For this review, use the dimensioned drawing (mm, ordinates from the lowest corner) and the shaded views. A direction names the side the tool comes from. Give positions to 0.01 mm unless a question says otherwise; leave off trailing zeros. Write each loop counter-clockwise with the first axis right and the second up, starting at its lowest first coordinate (ties: lowest second). Pieces come first, ordered by that corner, then holes.
1) Machinability: for the marked faces 4 and 5, which of the approach directions +Z, -Z, +X, -X, +Y, -Y give a long, thin tool a straight path to every point of the face, cutting with its end or side? Answer none if there is none.
2) Draft analysis for pull direction Z (two halves, no side actions). For the marked faces 1, 2 and 3, state which applies: pulls with the +Z half, pulls with the -Z half, needs draft (parallel to the pull), parting line crosses it, or undercut.
3) We need section D-D on z = 39.5. Give the boundary of the cut face in (x, y), and give its area (3 significant figures).
4) We need section A-A on z = 25. Give the boundary of the cut face in (x, y).
5) For P1, Ø8, axis at x = 18, y = 72, coming from the +Z side; P2, Ø6, axis at y = 26.5, z = 24, coming from the +X side; P3, Ø10, axis at x = 30.5, y = 20.5, coming from the -Z side (3 decimals); P4, Ø3, axis at x = 10.5, y = 17.5, coming from the -Z side, all flat-tipped, find the tip position at first contact; note any pin that passes through.
6) Wall thickness on line 1 along Y through (x, z) = (15, 25); line 2 along Z through (x, y) = (37, 40); line 3 along Y through (x, z) = (22.5, 15): over which ranges is each line inside the solid? List them lowest first.
7) We need section B-B on x = 25. Give the boundary of the cut face in (y, z), and give its area (3 significant figures).
8) We need section C-C on y = 40. Give the boundary of the cut face in (x, z).
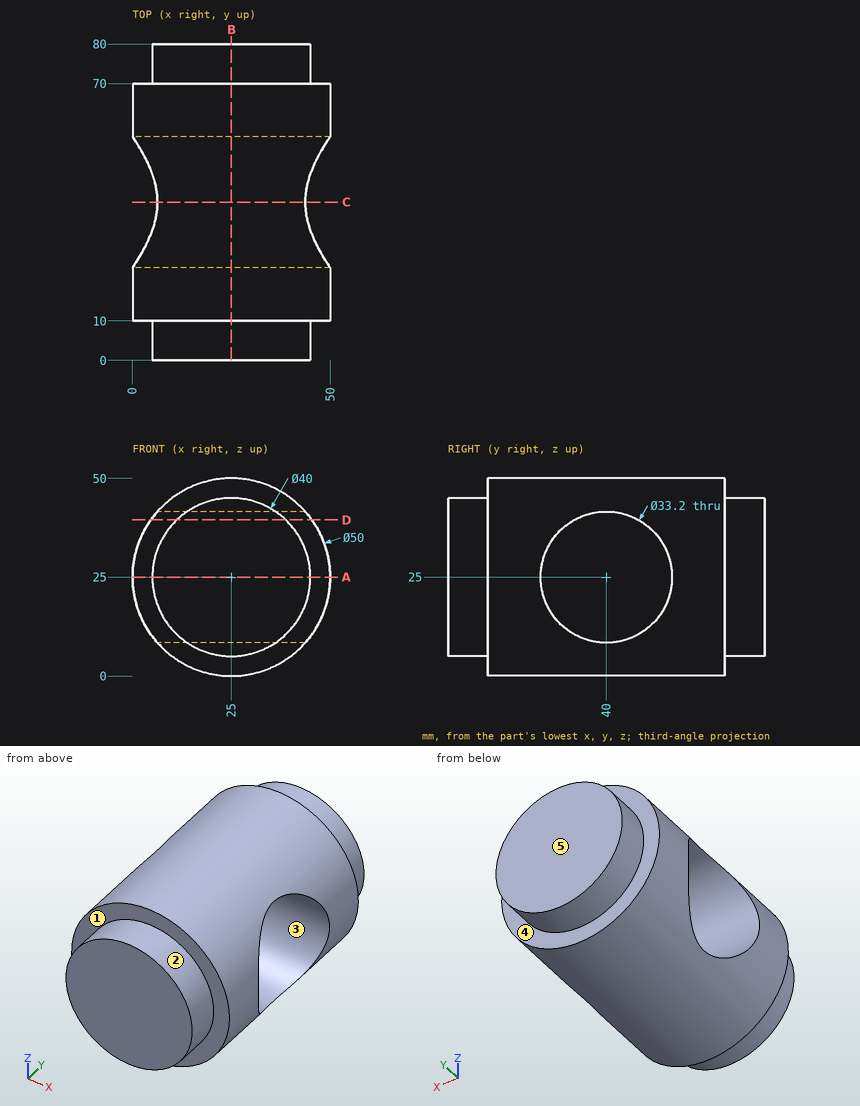
Results list:
1. face 4: +Y
1. face 5: +Z, -Z, +X, -X, +Y
2. face 1: needs draft
2. face 2: parting line crosses it
2. face 3: undercut
3. outline: (4.63, 10) - (11.23, 10) - (11.23, 0) - (38.77, 0) - (38.77, 10) - (45.37, 10) - (45.37, 31.92) - (4.63, 31.92) - close; (4.63, 48.08) - (45.37, 48.08) - (45.37, 70) - (38.77, 70) - (38.77, 80) - (11.23, 80) - (11.23, 70) - (4.63, 70) - close
3. area: 2,340 mm2
4. outline: (0, 10) - (5, 10) - (5, 0) - (45, 0) - (45, 10) - (50, 10) - (50, 23.4) - (0, 23.4) - close; (0, 56.6) - (50, 56.6) - (50, 70) - (45, 70) - (45, 80) - (5, 80) - (5, 70) - (0, 70) - close
5. P1: stops at z = 49.75
5. P2: passes through
5. P3: stops at z = 0.005
5. P4: stops at z = 3.65
6. line 1: y = 0 to 23.4, 56.6 to 80
6. line 2: z = 3.07 to 8.4, 41.6 to 46.93
6. line 3: y = 0 to 26.75, 53.25 to 80
7. outline: (0, 5) - (10, 5) - (10, 0) - (70, 0) - (70, 5) - (80, 5) - (80, 45) - (70, 45) - (70, 50) - (10, 50) - (10, 45) - (0, 45) - close; hole circle Ø33.2 at (40, 25)
7. area: 2,930 mm2
8. outline: (6.31, 8.4) arc R25 ccw to (43.69, 8.4) - close; (6.31, 41.6) - (43.69, 41.6) arc R25 ccw to start
